Input: part model. Units: mm. Frame: model coordinates. A direction names the side the tool comes from. Give positions to 0.01 mm unless a question says otherwise; leave off trailing zeros. Write each loop counter-clockwise with the first axis right and the second up, starting at its lowest first coordinate (ties: lowest second). Pieces come first, ordered by that corner, then holes. Notation, with made-up numbers: (2, -31.5) - (45, -31.5) arc R13 cw to (45, -20.5) - close; hole circle Ø11 at (-27, 82.25). An arc over 180 degrees is marked (long way). Answer as CSV lines item,"result".
```python
from build123d import *

# Parameters (mm, degrees)
SKETCH1_R           = 12
SKETCH1_R_2         = 1.75
BOSS_EXTRUDE1_DEPTH = 2.5
CUT_EXTRUDE3_DEPTH  = 2.5
SKETCH4_R           = 1.25
CUT_EXTRUDE4_DEPTH  = 5
SKETCH2_R           = 3
SKETCH2_R_2         = 1.75
BOSS_EXTRUDE2_DEPTH = 6


with BuildPart() as part:
    # Sketch1 → Boss-Extrude1 (new body)
    with BuildSketch(Plane(origin=(0, 0, 0), x_dir=(1, 0, 0), z_dir=(0, 1, 0))):
        Circle(SKETCH1_R)
        Circle(SKETCH1_R_2, mode=Mode.SUBTRACT)
    extrude(amount=BOSS_EXTRUDE1_DEPTH)

    # Sketch3 → Cut-Extrude3 (cut)
    with BuildSketch(Plane.XZ):
        Polygon((-5.161329605, 1.721273866), (-8.071331697, 3.318997608), (-10.910002092, 1.597723742), (-10.838670395, -1.721273866), (-7.928668303, -3.318997608), (-5.089997908, -1.597723742), align=None)
        Polygon((5.161329605, -1.721273866), (8.071331697, -3.318997608), (10.910002092, -1.597723742), (10.838670395, 1.721273866), (7.928668303, 3.318997608), (5.089997908, 1.597723742), align=None)
    extrude(amount=-CUT_EXTRUDE3_DEPTH, mode=Mode.SUBTRACT)

    # Sketch4 → Cut-Extrude4 (cut)
    with BuildSketch(Plane(origin=(0, 2.5, 0), x_dir=(1, 0, 0), z_dir=(0, 1, 0))):
        with Locations((0, 9)):
            Circle(SKETCH4_R)
        with Locations((0, 12)):
            Circle(SKETCH4_R)
    extrude(amount=-CUT_EXTRUDE4_DEPTH, mode=Mode.SUBTRACT)

    # Sketch2 → Boss-Extrude2 (add)
    with BuildSketch(Plane(origin=(0, 2.5, 0), x_dir=(1, 0, 0), z_dir=(0, 1, 0))):
        Circle(SKETCH2_R)
        Circle(SKETCH2_R_2, mode=Mode.SUBTRACT)
    extrude(amount=BOSS_EXTRUDE2_DEPTH)

    # Mirror7: part across plane


with BuildPart() as part_1:
    add(part.part)
    add(part.part.mirror(Plane.ZX.offset(8.5)))


solid = part_1.part
```
Item 1: Cut plane A-A on y = 16. Return the cut outline in (x, z).
The answers:
outline,"(-1.25, -11.93) arc R1.25 cw to (1.25, -11.93) arc R12 ccw (long way) to start; hole (-10.91, 1.6) - (-10.84, -1.72) - (-7.93, -3.32) - (-5.09, -1.6) - (-5.16, 1.72) - (-8.07, 3.32) - close; hole circle Ø3.5 at (0, 0); hole circle Ø2.5 at (0, -9); hole (5.09, 1.6) - (5.16, -1.72) - (8.07, -3.32) - (10.91, -1.6) - (10.84, 1.72) - (7.93, 3.32) - close"
Item 2: Cut plane C-C on x = -4. Return the cut outline in (y, z).
The answers:
outline,"(0, -11.31) - (2.5, -11.31) - (2.5, 11.31) - (0, 11.31) - close; (14.5, -11.31) - (17, -11.31) - (17, 11.31) - (14.5, 11.31) - close"
Item 3: Cut plane B-B on x = 0. Return the cut outline in (y, z), plus the area to 3 significant figures.
The answers:
outline,"(0, -10.75) - (2.5, -10.75) - (2.5, -10.25) - (0, -10.25) - close; (0, -7.75) - (2.5, -7.75) - (2.5, -3) - (14.5, -3) - (14.5, -7.75) - (17, -7.75) - (17, -1.75) - (0, -1.75) - close; (0, 1.75) - (17, 1.75) - (17, 12) - (14.5, 12) - (14.5, 3) - (2.5, 3) - (2.5, 12) - (0, 12) - close; (14.5, -10.75) - (17, -10.75) - (17, -10.25) - (14.5, -10.25) - close"
area,"114 mm²"
Item 4: Contact query for flat-ended pins moving along their axis: pin 1 (4 mm diameter, centred on y = 8, z = 3, fed in from -X); pin 2 (1 mm diameter, centred on y = 2, z = -1, fed in from +X). Output: stop coordinate, or through.
The answers:
pin 1,"x = -2.83"
pin 2,"x = 11.99"
Item 5: Cut plane D-D on z = -5.5. Return the cut outline in (x, y), plus the area to 3 significant figures.
The answers:
outline,"(-10.67, 0) - (10.67, 0) - (10.67, 2.5) - (-10.67, 2.5) - close; (-10.67, 14.5) - (10.67, 14.5) - (10.67, 17) - (-10.67, 17) - close"
area,"107 mm²"
Item 6: Mould query, pull axis Z, two halves, no side actions, for faces 3 (the face through (-0.16, 15.73, -10.24)), 4 (the face through (-0.51, 1.23, 11.99)), 5 (the face through (2, 2.5, 3)). Classes: +Z half, -Z half, draft (parallel to the pull), parting line (faces both ways), or undercut.
The answers:
face 3,"undercut"
face 4,"parting line"
face 5,"draft"
Item 7: Ray query, line 1 (Z direction, x = 0, y = 1.5); line 2 (Y direction, x = 1.5, z = -7); line 3 (Z direction, x = 0, y = 6.75). Return the intervals inside material, ascending. Write a range as from..to.
The answers:
line 1,"-10.75..-10.25, -7.75..-1.75, 1.75..12"
line 2,"0..2.5, 14.5..17"
line 3,"-3..-1.75, 1.75..3"
Item 8: Reachability of faces 1 (the face through (0, 0, 3)), 2 (the face through (6.53, 1.23, 2.47)) from +Z, -Z, +X, -X, +Y, -Y: full face, straight path, thin tool, end or side. Return the list, or none.
The answers:
face 1,"+Z, -Z, +X, -X, -Y"
face 2,"+Y, -Y"
